Source: three-view drawing plus pictorial views. Frame: mm from the lowest corner of the part. Give positions to 0.01 mm unless a question says otherwise; leave off trailing zeros. Loops run counter-clockwise (first coordinate to the right, second up) from the corner with the lowest first, then second, coordinate; pieces in that order, holes last. Notation, with made-up numbers: (6, 83) -> (28, 83) arc R24 cw to (28, 94) -> close; hole circle Ø5 at (69.25, 76.25). An arc over 180 degrees is marked (long way). One line per item, written item: value. Start each with the question number.
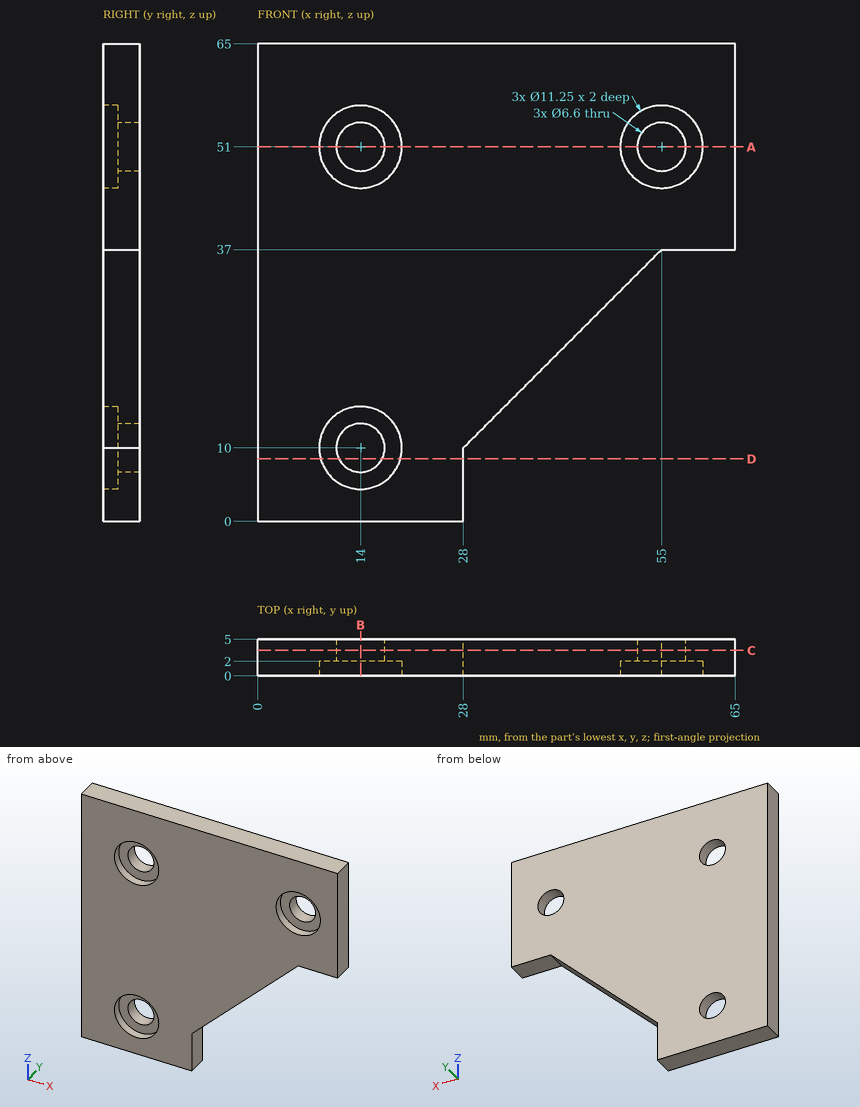
Item 1: Ray query, line 1 along Z through (x, y) = (14, 3.3); line 2 along Z through (x, y) = (14, 0.6) (3 decimals); line 3 along Z through (x, y) = (55, 3.9). Return the intervals inside material, ascending. Write a range as [from, to].
Item 2: Section A-A, the plane z = 51. Output: boundary loops of the cut face in (x, y) (3 decimals), then the cut area to 3 significant figures.
Item 3: Section B-B, the plane x = 14. Output: boundary loops of the cut face in (y, z) (3 decimals), then the cut area to 3 significant figures.
Item 4: Pin query (flat end, axial travel): pin 1 (5.5 mm diameter, centred on x = 56.5, z = 49, fed in from -Y); pin 2 (4 mm diameter, centred on x = 17.5, z = 54.5, fed in from -Y); pin 3 (1.5 mm diameter, centred on y = 1.5, z = 5.5, fed in from +X); pin 4 (5.5 mm diameter, centred on x = 14, z = 10, fed in from -Y). Return the tip coordinate at first contact, or that it passes through.
Item 5: Section C-C, the plane y = 3.5. Output: boundary loops of the cut face in (x, z), then the cut area to 3 significant figures.
Item 6: Section D-D, the plane z = 8.5. Output: boundary loops of the cut face in (x, y), then the cut area to 3 significant figures.
Geometry check:
1. line 1: z = [0, 6.7], [13.3, 47.7], [54.3, 65]
1. line 2: z = [0, 4.375], [15.625, 45.375], [56.625, 65]
1. line 3: z = [37, 47.7], [54.3, 65]
2. outline: (0, 0) -> (8.375, 0) -> (8.375, 2) -> (10.7, 2) -> (10.7, 5) -> (0, 5) -> close; (17.3, 2) -> (19.625, 2) -> (19.625, 0) -> (49.375, 0) -> (49.375, 2) -> (51.7, 2) -> (51.7, 5) -> (17.3, 5) -> close; (58.3, 2) -> (60.625, 2) -> (60.625, 0) -> (65, 0) -> (65, 5) -> (58.3, 5) -> close
2. area: 240 mm2
3. outline: (0, 0) -> (5, 0) -> (5, 6.7) -> (2, 6.7) -> (2, 4.375) -> (0, 4.375) -> close; (0, 15.625) -> (2, 15.625) -> (2, 13.3) -> (5, 13.3) -> (5, 47.7) -> (2, 47.7) -> (2, 45.375) -> (0, 45.375) -> close; (0, 56.625) -> (2, 56.625) -> (2, 54.3) -> (5, 54.3) -> (5, 65) -> (0, 65) -> close
3. area: 240 mm2
4. pin 1: stops at y = 2
4. pin 2: stops at y = 0
4. pin 3: stops at x = 28
4. pin 4: passes through
5. outline: (0, 0) -> (28, 0) -> (28, 10) -> (55, 37) -> (65, 37) -> (65, 65) -> (0, 65) -> close; hole circle Ø6.6 at (14, 10); hole circle Ø6.6 at (14, 51); hole circle Ø6.6 at (55, 51)
5. area: 3,120 mm2
6. outline: (0, 0) -> (8.58, 0) -> (8.58, 2) -> (11.06, 2) -> (11.06, 5) -> (0, 5) -> close; (16.94, 2) -> (19.42, 2) -> (19.42, 0) -> (28, 0) -> (28, 5) -> (16.94, 5) -> close
6. area: 101 mm2
